Verification items for the finished model (mm, model axes). A direction names the side the tool comes from. Coordinates: 2 decimals unless noted, no trailing zeros. Write item = value, one per line. Start each with the question number.
(1) Section check A-A (x = 0). State how many separate pieces and enclosed holes the cut face has, plus the area to 3 significant figures.
(2) Set-up check for faces 1 (the face through (-38.481, -12.445, 4.696)), 2 (the face through (59.28, -6.23, 4.43)), 3 (the face through (-39.369, 2.625, 5.888)): record each of +Z, -Z, +X, -X, +Y, -Y from which the full face is reachable in a straight line by a thin tool's end or side.
(3) Gauge pin test, flat ends, axial feed: pin 1 Ø5 at (x, z) = (-6, 2.5) entering from -Y; pin 2 Ø1.5 at (x, z) = (0, 4.5) entering from +Y; pin 3 Ø12.5 at (x, y) = (10, -50) entering from +Z (3 decimals); pin 4 Ø1 at (y, z) = (44, 8) entering from -X. Record the tip position at first contact, or that the pin passes through.
(4) Material ranges on probe 1 along Y at (x, z) = (-21, 3.75); probe 2 along Y at (x, z) = (-2, 1.5); probe 3 along X at (y, z) = (-23.5, 1.75), recorded low to high. Write a range as [from, to].
```python
from build123d import *

# Parameters (mm, degrees)
SKETCH1_R                = 66.4845
BOSS_EXTRUDE1_DEPTH      = 9.525
CUT_EXTRUDE1_DEPTH       = 95.504513678
FILLET1_R                = 6.35
SKETCH3_W                = 41.453999896
SKETCH3_H                = 21.463
CUT_EXTRUDE5_DEPTH       = 3.175
SKETCH4_W                = 31.293999896
SKETCH4_H                = 16.383
CUT_EXTRUDE6_DEPTH       = 95.237465907
FILLET2_R                = 2.54
CIRPATTERN1_COUNT        = 5
FILLET2_OF_CIRPATTERN1_R = 2.54


with BuildPart() as part:
    # Sketch1 → Boss-Extrude1 (new body)
    with BuildSketch(Plane.XY):
        with Locations(Location((0, 0, 0), (0, 0, 180))):
            Circle(SKETCH1_R)
    extrude(amount=BOSS_EXTRUDE1_DEPTH)

    # Sketch2 → Cut-Extrude1 (cut, through all)
    with BuildSketch(Plane.XY.offset(9.525)):
        Polygon((24.653254911, 33.93229434), (-24.653254911, 33.93229434), (-39.889804379, -12.960983122), (0, -41.942622437), (39.889804379, -12.960983122), align=None)
    extrude(amount=-CUT_EXTRUDE1_DEPTH, mode=Mode.SUBTRACT)

    # Fillet1
    fillet1_edges = [part.edges().sort_by_distance(p)[0] for p in [
        (24.653254911, 33.93229434, 4.7625),
        (39.889804379, -12.960983122, 4.7625),
        (0, -41.942622437, 4.7625),
        (-39.889804379, -12.960983122, 4.7625),
        (-24.653254911, 33.93229434, 4.7625),
    ]]
    fillet(fillet1_edges, radius=FILLET1_R)

    # Sketch3 → Cut-Extrude5 (cut)
    with BuildSketch(Plane.XY.offset(9.525)):
        Polygon((16.110904278, 40.793694229), (16.110904278, 59.716694229), (38.633115128, 47.973184599), align=None)
        with Locations((-9.37859567, 48.985194229)):
            Rectangle(SKETCH3_W, SKETCH3_H)
    cut_extrude5 = extrude(amount=-CUT_EXTRUDE5_DEPTH, mode=Mode.SUBTRACT)

    # Sketch4 → Cut-Extrude6 (cut, through all)
    with BuildSketch(Plane.XY.offset(6.35)):
        with Locations((-9.37859567, 46.445194229)):
            Rectangle(SKETCH4_W, SKETCH4_H)
    cut_extrude6 = extrude(amount=-CUT_EXTRUDE6_DEPTH, mode=Mode.SUBTRACT)

    # Fillet2
    fillet2_edges = [part.edges().sort_by_distance(p)[0] for p in [
        (27.372009703, 44.383439414, 6.35),
        (16.110904278, 50.255194229, 6.35),
        (27.372009703, 53.844939414, 6.35),
        (-25.025595618, 38.253694229, 3.175),
        (-25.025595618, 54.636694229, 3.175),
        (6.268404278, 54.636694229, 3.175),
        (6.268404278, 38.253694229, 3.175),
    ]]
    fillet(fillet2_edges, radius=FILLET2_R)

    # Sketch7 → #44 (0.086) Diameter Hole1 (revolve, cut)
    with BuildSketch(Plane(origin=(28.097563823, 60.255420067, 4.7625), x_dir=(-0.9063077870366496, 0.4226182617407002, 0), z_dir=(0, 0, 1))):
        Polygon((0, 0), (0, 14.626259968), (1.0922, 13.97), (1.0922, 0), align=None)
    f_44_0_086_diameter_hole1 = revolve(axis=Axis((30.781189785, 66.010474515, 4.7625), (-0.42261826174070033, -0.9063077870366496, 0)), mode=Mode.SUBTRACT)

    # CirPattern1: Cut-Extrude5, Cut-Extrude6, #44 (0.086) Diameter Hole1 ×5 about axis
    cirpattern1_axis = Axis((0, 0, 0), (0, 0, 1))
    add([cut_extrude5.rotate(cirpattern1_axis, i * 360 / CIRPATTERN1_COUNT) for i in range(1, CIRPATTERN1_COUNT)], mode=Mode.SUBTRACT)
    add([cut_extrude6.rotate(cirpattern1_axis, i * 360 / CIRPATTERN1_COUNT) for i in range(1, CIRPATTERN1_COUNT)], mode=Mode.SUBTRACT)
    add([f_44_0_086_diameter_hole1.rotate(cirpattern1_axis, i * 360 / CIRPATTERN1_COUNT) for i in range(1, CIRPATTERN1_COUNT)], mode=Mode.SUBTRACT)

    # Fillet2 of CirPattern1
    fillet2_of_cirpattern1_edges = [part.edges().sort_by_distance(p)[0] for p in [
        (-33.752743102, 39.74756524, 6.35),
        (-42.816986733, 30.852089569, 6.35),
        (-42.751164331, 42.671329532, 6.35),
        (-44.114759509, -11.979714172, 3.175),
        (-59.695918416, -6.917088753, 3.175),
        (-50.025540626, 22.845273769, 3.175),
        (-34.44438172, 17.78264835, 3.175),
        (-48.232352153, -19.818093126, 6.35),
        (-42.573257375, -31.187554251, 6.35),
        (-53.793682318, -27.472607418, 6.35),
        (-2.238825164, -45.657564763, 3.175),
        (-11.868510953, -58.911690182, 3.175),
        (-37.18588869, -40.517538558, 3.175),
        (-27.556202902, -27.263413139, 3.175),
        (3.943510114, -51.995820384, 6.35),
        (16.505266663, -50.127058123, 6.35),
        (9.504840278, -59.650334676, 6.35),
        (42.731089463, -16.238212695, 3.175),
        (52.360775251, -29.492338114, 3.175),
        (27.043397513, -47.886489738, 3.175),
        (17.413711725, -34.632364319, 3.175),
        (50.669575439, -12.317091144, 6.35),
        (52.774073166, 0.207328575, 6.35),
        (59.667996668, -9.393326852, 6.35),
        (28.648090829, 35.621797401, 3.175),
        (44.229249735, 40.68442282, 3.175),
        (53.899627525, 10.922060298, 3.175),
        (38.318468619, 5.859434879, 3.175),
    ]]
    fillet(fillet2_of_cirpattern1_edges, radius=FILLET2_OF_CIRPATTERN1_R)


solid = part.part
```
Response:
q1.separate_pieces = 3
q1.enclosed_holes = 0
q1.area = 365 mm2
q2.face_1 = +Z, -Z
q2.face_2 = none
q2.face_3 = +Z
q3.pin_1 = -66.39
q3.pin_2 = 66.48
q3.pin_3 = 9.525
q3.pin_4 = -50.28
q4.probe_1 = [-63.08, -52.28], [-32.03, -26.69], [33.86, 38.25], [54.64, 63.08]
q4.probe_2 = [-66.45, -40.12], [33.93, 38.25], [54.64, 66.45]
q4.probe_3 = [-62.19, -25.38], [25.38, 32.74], [48.01, 62.19]
